from build123d import *

# Parameters (mm, degrees)
BOSS_EXTRUDE1_DEPTH = 2


with BuildPart() as part:
    # Sketch1 → Boss-Extrude1 (new body)
    with BuildSketch(Plane.XY):
        with BuildLine():
            Line((-5, 0), (-5, -27))
            ThreePointArc((-5, -27), (-4.121320344, -29.121320344), (-2, -30))
            Line((-2, -30), (2, -30))
            ThreePointArc((2, -30), (4.121320344, -29.121320344), (5, -27))
            Line((5, -27), (5, 0))
            ThreePointArc((5, 0), (0, 5), (-5, 0))
        make_face()
        with BuildLine():
            Line((-1.322875656, 1.5), (1.322875656, 1.5))
            ThreePointArc((1.322875656, 1.5), (0, -2), (-1.322875656, 1.5))
        make_face(mode=Mode.SUBTRACT)
    extrude(amount=BOSS_EXTRUDE1_DEPTH)


solid = part.part
Source: CAD feature listing. Evaluate the final solid. Frame: model axes, mm. A direction names the side the tool comes from. Give positions to 0.01 mm unless a question says otherwise; leave off trailing zeros. Order: outer loops, then holes, each group sorted by start corner. A loop starts at its lowest first (then second) coordinate and runs counter-clockwise, first axis right, second up. Notation, with made-up numbers: (75, 85.5) -> (124, 85.5) arc R16 cw to (124, 106.5) -> close; hole circle Ø1 at (-6, 15). An arc over 180 degrees is marked (long way). Write item = value, one per line.
Q1. Cut plane A-A, the plane z = 0.6. Output: boundary loops of the cut face in (x, y).
Data:
outline = (-5, -27) arc R3 ccw to (-2, -30) -> (2, -30) arc R3 ccw to (5, -27) -> (5, 0) arc R5 ccw to (-5, 0) -> close; hole (-1.32, 1.5) arc R2 ccw (long way) to (1.32, 1.5) -> close
Q2. Pin query (flat end, axial travel): pin 1 (2.5 mm diameter, centred on x = 0, y = 0, fed in from +Z). Return the tip coordinate at first contact, or that it passes through.
Data:
pin_1 = through
Q3. Material intervals for line 1 (Y direction, x = 1.5, z = 0.4); line 2 (Y direction, x = -3.25, z = 1.75); line 3 (Y direction, x = -1, z = 1.3), sorted ascending. Write a range as from..to.
Data:
line_1 = -30..-1.32, 1.32..4.77
line_2 = -29.73..3.8
line_3 = -30..-1.73, 1.5..4.9
Q4. Pull-direction query (X, two-part tool) for faces 1 (the face through (-5, -13, 1)), 2 (the face through (0, -2, 1)), 3 (the face through (4.1, -29.14, 0.99)); classes: released by +X, released by -X, zero draft, split by the parting line, or undercut.
Data:
face_1 = released by -X
face_2 = undercut
face_3 = released by +X
Q5. Cut plane C-C, the plane x = 2.5. Output: boundary loops of the cut face in (y, z).
Data:
outline = (-29.96, 0) -> (4.33, 0) -> (4.33, 2) -> (-29.96, 2) -> close
Q6. Set-up query: faces 4 (the face through (0, 1.5, 1)), 5 (the face through (0, -12, 0)). Return all of +Z, -Z, +X, -X, +Y, -Y with unobstructed straight access to the full face (end or side cutting, diameter ignored); none if empty.
Data:
face_4 = +Z, -Z
face_5 = -Z, +X, -X, +Y, -Y
Q7. Cut plane B-B, the plane x = 0. Output: boundary loops of the cut face in (y, z), and give its area (3 significant figures).
Data:
outline = (-30, 0) -> (-2, 0) -> (-2, 2) -> (-30, 2) -> close; (1.5, 0) -> (5, 0) -> (5, 2) -> (1.5, 2) -> close
area = 63.0 mm^2
Q8. Cut plane D-D, the plane x = -3. Output: boundary loops of the cut face in (y, z).
Data:
outline = (-29.83, 0) -> (4, 0) -> (4, 2) -> (-29.83, 2) -> close
